Check sheet for the modelled part. Datum: model origin and axes. Units: mm. A direction names the side the tool comes from. Give positions to 0.01 mm unless a question says otherwise; leave off trailing zeros. Loops run counter-clockwise (first coordinate to the right, second up) from the corner with the lowest first, then second, coordinate; pieces in that order, holes last. Notation, with made-up numbers: M 63,65.25 L 118,65.25 A6 ccw 118,74.25 Z; hole C 64.25,50 d1. An arc over 180 degrees is marked long. Write each question's results on one line, items separated by ' | '. Start each with the question number.
1. Sectioned sample at C-C on z = 7. Record the cut outline in (x, y), and give its area (3 significant figures).
2. Draft check along Z on faces 3 (the cylindrical face through (2.58, 4.05, 4.45)), 4 (the flat face through (0, 2, 0)), 5 (the flat face through (0, 2, 9)), 6 (the cylindrical face through (-5.158, -3.955, 0.493)). Enter one of: pulls with the +Z half, pulls with the -Z half, needs draft (parallel to the pull), parting line crosses it, or undercut.
3. Tool access check on faces 1 (the cylindrical face through (-1.5, 0.07, 4.44)), 2 (the flat face through (-1, -5, 1)). Record the directions out of +Z, -Z, +X, -X, +Y, -Y that give a thin tool (end or side, any length) a straight path to the whole face; none if there is none.
4. Go/stop test with flat-tipped pins: pin 1 (2 mm diameter, centred on y = -3, z = 8, fed in from +X); pin 2 (3 mm diameter, centred on x = -1.5, z = 4, fed in from +Y); pin 3 (3 mm diameter, centred on x = -5, z = 5.5, fed in from +Y); pin 4 (1.8 mm diameter, centred on x = 0, y = 0, fed in from -Z). Record where each tip stops, or that it passes through.
5. Sectioned sample at A-A on x = 0. Record the cut outline in (y, z), and give its area (3 significant figures).
6. Material ranges on line 1 along Z through (x, y) = (-3.5, -4.5); line 2 along Y through (x, z) = (0, 2.75); line 3 along Y through (x, z) = (-1, 7.75), recorded low to high.
7. Sectioned sample at D-D on x = -2. Record the cut outline in (y, z), and give its area (3 significant figures).
```python
from build123d import *

# Parameters (mm, degrees)
SKETCH1_R           = 6.5
SKETCH1_R_2         = 1.5
BOSS_EXTRUDE1_DEPTH = 1
SKETCH2_R           = 4.8
SKETCH2_R_2         = 1.5
BOSS_EXTRUDE2_DEPTH = 7
SKETCH3_R           = 6.5
SKETCH3_R_2         = 1.5
BOSS_EXTRUDE3_DEPTH = 1


with BuildPart() as part:
    # Sketch1 → Boss-Extrude1 (new body)
    with BuildSketch(Plane.XY):
        Circle(SKETCH1_R)
        Circle(SKETCH1_R_2, mode=Mode.SUBTRACT)
    extrude(amount=BOSS_EXTRUDE1_DEPTH)

    # Sketch2 → Boss-Extrude2 (add)
    with BuildSketch(Plane.XY.offset(1)):
        Circle(SKETCH2_R)
        Circle(SKETCH2_R_2, mode=Mode.SUBTRACT)
    extrude(amount=BOSS_EXTRUDE2_DEPTH)

    # Sketch3 → Boss-Extrude3 (add)
    with BuildSketch(Plane.XY.offset(8)):
        Circle(SKETCH3_R)
        Circle(SKETCH3_R_2, mode=Mode.SUBTRACT)
    extrude(amount=BOSS_EXTRUDE3_DEPTH)


solid = part.part
```
Output values:
1) outline: C 0,0 d9.6; hole C 0,0 d3 | area: 65.3 mm2
2) face 3: undercut | face 4: pulls with the -Z half | face 5: pulls with the +Z half | face 6: needs draft
3) face 1: +Z, -Z | face 2: none
4) pin 1: x = 6.18 | pin 2: y = 4.8 | pin 3: y = 3.28 | pin 4: through
5) outline: M -6.5,0 L -1.5,0 L -1.5,9 L -6.5,9 L -6.5,8 L -4.8,8 L -4.8,1 L -6.5,1 Z; M 1.5,0 L 6.5,0 L 6.5,1 L 4.8,1 L 4.8,8 L 6.5,8 L 6.5,9 L 1.5,9 Z | area: 66.2 mm2
6) line 1: 0 to 1, 8 to 9 | line 2: -4.8 to -1.5, 1.5 to 4.8 | line 3: -4.69 to -1.12, 1.12 to 4.69
7) outline: M -6.18,0 L 6.18,0 L 6.18,1 L 4.36,1 L 4.36,8 L 6.18,8 L 6.18,9 L -6.18,9 L -6.18,8 L -4.36,8 L -4.36,1 L -6.18,1 Z | area: 85.8 mm2
